The drawing under review shows one solid part. Ordinate dimensions are in mm from its lowest x, y, z. A direction names the side the tool comes from. Coordinates: 2 decimals unless noted, no trailing zeros. Order: outer loops, then holes, each group sorted by start corner. A loop starts at its lowest first (then second) coordinate and runs counter-clockwise, first axis right, second up. Notation, with made-up numbers: M 26,89.25 L 34,89.25 A13 ccw 34,102.25 Z; hole C -14,76 d11. An arc over 180 degrees is marked long. Answer as a JSON object with one key per item and string values.
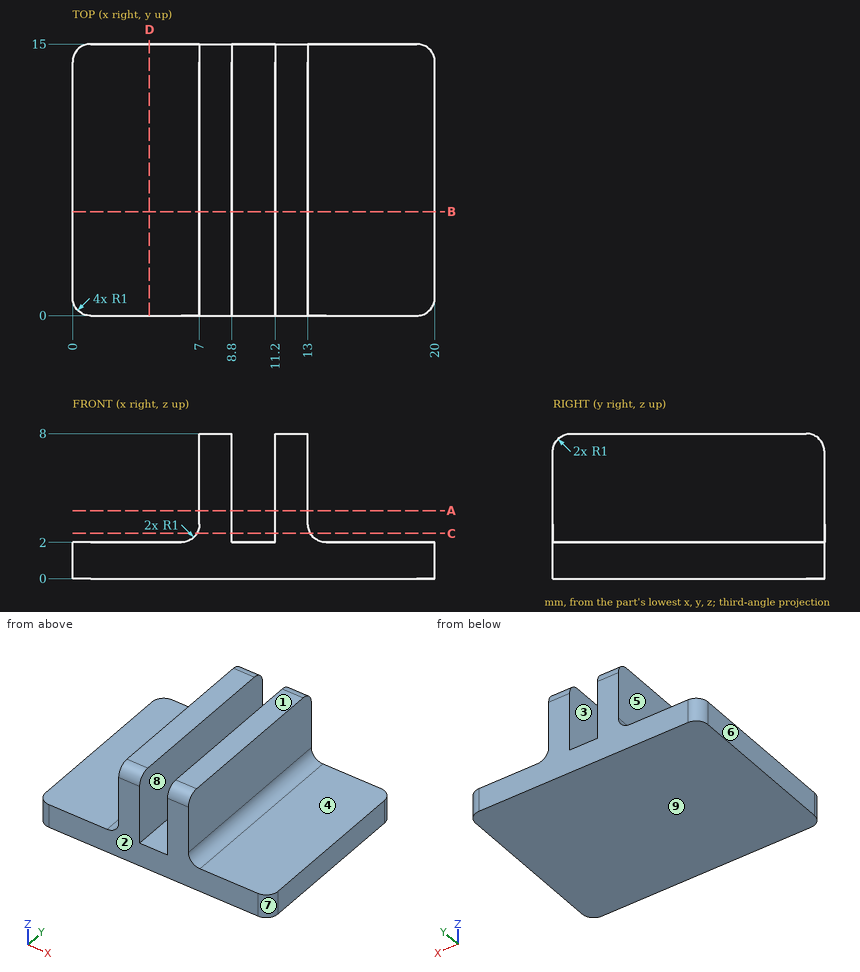
1) Insertion check: pin 1 Ø1.8 at (x, y) = (2.5, 4) entering from +Z; pin 2 Ø3 at (y, z) = (9.5, 4.5) entering from -X; pin 3 Ø1.5 at (y, z) = (8.5, 5) entering from +X. Each pin has a flat end and moves straight along its axis. Give the tip position at first contact, or say it passes through.
Taken from the geometry:
{"pin 1": "stops at z = 2", "pin 2": "stops at x = 7", "pin 3": "stops at x = 13"}
2) Add section C-C (z = 2.5). State the section outline as (x, y) points.
Taken from the geometry:
{"outline": "M 6.87,0 L 8.8,0 L 8.8,15 L 6.87,15 Z; M 11.2,0 L 13.13,0 L 13.13,15 L 11.2,15 Z"}
3) Tool access review of the marked faces 1, 2, 3, 4 and 5: name each direction out of +Z, -Z, +X, -X, +Y, -Y from which nothing blocks a thin tool from reaching the whole face with its end or side.
Taken from the geometry:
{"face 1": "+Z, +X, -X, +Y, -Y", "face 2": "+Z, -Z, +X, -X, -Y", "face 3": "+Z, +Y, -Y", "face 4": "+Z, +X, +Y, -Y", "face 5": "+Z, -X, +Y, -Y"}
4) Add section B-B (y = 5.75). State the section outline as (x, z) points, and give its area (3 significant figures).
Taken from the geometry:
{"outline": "M 0,0 L 20,0 L 20,2 L 14,2 A1 cw 13,3 L 13,8 L 11.2,8 L 11.2,2 L 8.8,2 L 8.8,8 L 7,8 L 7,3 A1 cw 6,2 L 0,2 Z", "area": "62.0 mm2"}
5) Add section A-A (z = 3.75). State the section outline as (x, y) points, and give its area (3 significant figures).
Taken from the geometry:
{"outline": "M 7,0 L 8.8,0 L 8.8,15 L 7,15 Z; M 11.2,0 L 13,0 L 13,15 L 11.2,15 Z", "area": "54.0 mm2"}
6) To check wall thickness, follow L1, parallel to X at y = 5.25, z = 3.5; L2, parallel to Z at x = 15, y = 5.5; L3, parallel to X at y = 3.75, z = 2.5. State the ranges of each line that lie inside material, in increasing order.
Taken from the geometry:
{"L1": "x = 7 to 8.8, 11.2 to 13", "L2": "z = 0 to 2", "L3": "x = 6.87 to 8.8, 11.2 to 13.13"}
7) Add section D-D (x = 4.25). State the section outline as (y, z) points.
Taken from the geometry:
{"outline": "M 0,0 L 15,0 L 15,2 L 0,2 Z"}
8) Mouldability with a two-part tool opening along X and no side actions: class the marked faces 6, 7, 8 and 9 as released by +X, released by -X, zero draft, split by the parting line, or undercut.
Taken from the geometry:
{"face 6": "released by -X", "face 7": "released by +X", "face 8": "undercut", "face 9": "zero draft"}
